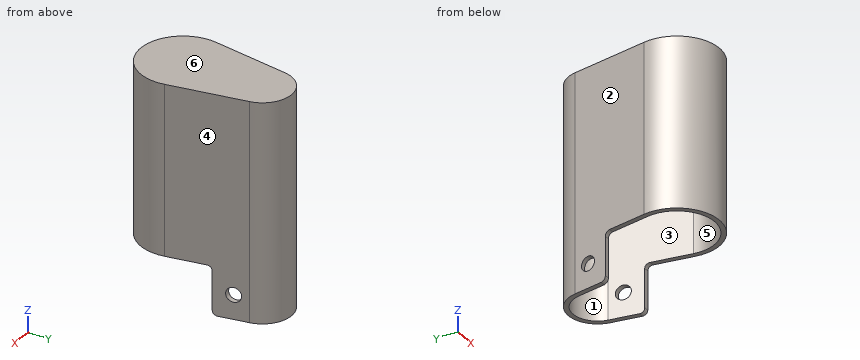
from build123d import *

# Parameters (mm, degrees)
F1_DEPTH = 57.15
F2_T     = -1.27
F3_W     = 24.3205
F3_H     = 12.7
F3_R     = 1.905
F4_DEPTH = 24.8444639078
F5_R     = 1.27


with BuildPart() as f1:
    # F0 (on Top) → F1 (new body)
    with BuildSketch(Plane.XY):
        with BuildLine():
            Line((6.2188556471, 34.2943200643), (2.7758060277, 14.0519526863))
            ThreePointArc((2.7758060277, 14.0519526863), (13.7309639078, 1.0760761619), (24.6861217879, 14.0519526863))
            Line((24.6861217879, 14.0519526863), (21.2430721684, 34.2943200643))
            ThreePointArc((21.2430721684, 34.2943200643), (13.7309639078, 40.6365761619), (6.2188556471, 34.2943200643))
        make_face()
    extrude(amount=F1_DEPTH)

    # F2
    f2_openings = [f1.faces().sort_by_distance(p)[0] for p in [
        (13.730964, 19.748404, 0),
    ]]
    offset(amount=F2_T, openings=f2_openings)

    # F3 (on Right) → F4 (cut, through all)
    with BuildSketch(Plane.YZ):
        with Locations((13.2363261619, 6.35)):
            Rectangle(F3_W, F3_H)
        with Locations((30.4765761619, 6.35)):
            Circle(F3_R)
    extrude(amount=F4_DEPTH, mode=Mode.SUBTRACT)

    # F5
    f5_edges = [f1.edges().sort_by_distance(p)[0] for p in [
        (5.349547, 25.396576, 12.7),
        (22.11238, 25.396576, 12.7),
        (5.349547, 25.396576, 0),
        (22.11238, 25.396576, 0),
        (13.730964, 2.346076, 55.88),
        (21.712579, 23.960179, 55.88),
        (13.730964, 39.366576, 55.88),
        (5.749349, 23.960179, 55.88),
    ]]
    fillet(f5_edges, radius=F5_R)


solid = f1.part
Read the model definition and answer for the solid it produces. Units are mm, in the model's axes. Face numbers are marked on the shaded views. A direction names the side the tool comes from. Coordinates: 2 decimals unless noted, no trailing zeros. Write each loop counter-clockwise with the first axis right and the second up, starting at its lowest first coordinate (ties: lowest second). Pieces come first, ordered by that corner, then holes. Notation, with made-up numbers: (33, 49) - (47, 49) arc R31 ccw to (47, 87) - close; hole circle Ø6 at (-7, 71). An arc over 180 degrees is marked (long way). One line per question, with ' | ' between items.
Q1. Each of these flat-tipped pins is pushed along its axis until it touches: P1, Ø3.5, axis at y = 30.48, z = 6.35, coming from the -X side; P2, Ø3, axis at x = 6.5, z = 16, coming from the -Y side; P3, Ø5, axis at x = 10.5, y = 24, coming from the -Z side; P4, Ø5, axis at y = 30.48, z = 6.35, coming from the +X side. Where does it stop, or does it pass through?
Result set:
P1: through | P2: y = 2.67 | P3: z = 55.88 | P4: x = 22.32
Q2. Consider L1, parallel to Z at x = 9.5, y = 7; L2, parallel to X at y = 24, z = 42; L3, parallel to X at y = 11.5, z = 32.5. Determine where each line is inside the solid, lowest interval first. Write a range as [from, to].
Result set:
L1: [55.88, 57.15] | L2: [4.47, 5.76], [21.71, 22.99] | L3: [2.64, 3.91], [23.55, 24.82]
Q3. For the marked faces 1 and 2, determine the directions among +Z, -Z, +X, -X, +Y, -Y from which every point of the face is accessible in a straight line to the end or side of a thin tool.
Result set:
face 1: -Z | face 2: +Z, -Z, -X, +Y
Q4. Determine the mould class of the marked faces 3, 4, 5 and 6 for opening direction Y: +Y half, -Y half, draft (parallel to the pull), parting line (faces both ways), or undercut.
Result set:
face 3: undercut | face 4: +Y half | face 5: undercut | face 6: draft
Q5. Find section A-A, the plane z = 10. Write down the section's boundary in (x, y).
Result set:
outline: (4.71, 25.4) - (5.99, 25.4) - (7.47, 34.08) arc R6.35 cw to (19.99, 34.08) - (21.47, 25.4) - (22.76, 25.4) - (21.24, 34.29) arc R7.62 ccw to (6.22, 34.29) - close
